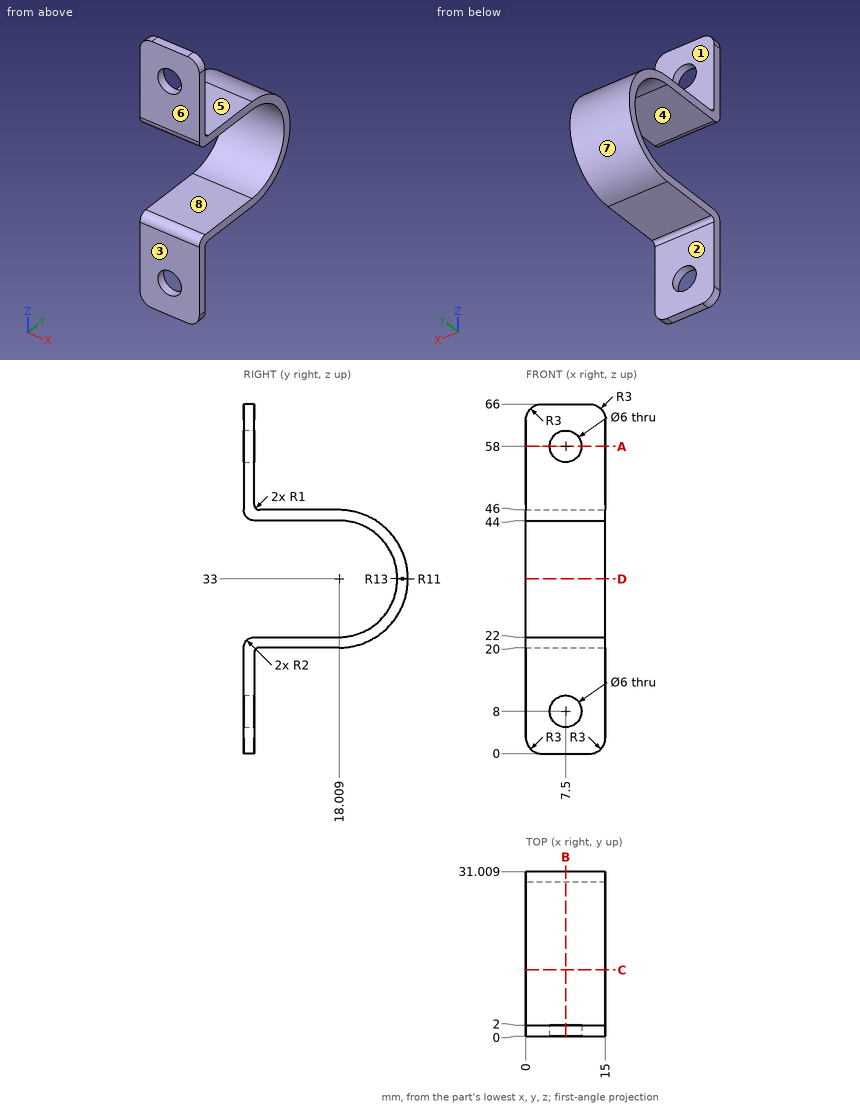
Study the drawing (mm; zero at the part's minimum x, y, z) and answer. A direction names the side the tool comes from. Round coordinates to 2 decimals unless told otherwise and drop trailing zeros. Order: outer loops, then holes, each group sorted by start corner. A loop starts at its lowest first (then second) coordinate and runs counter-clockwise, first axis right, second up. Notation, with made-up numbers: M 41.5,39 L 98.5,39 A30 ccw 98.5,61 Z; hole C -38.75,-40 d8. An arc over 180 degrees is marked long. One line per item, written item: value.
Q1. Flat-ended cylindrical pins translate along their axes: pin 1 (3 mm diameter, centred on x = 1.5, z = 57.5, fed in from +Y); pin 2 (1.5 mm diameter, centred on x = 4, y = 22.5, fed in from -Z); pin 3 (5 mm diameter, centred on x = 10, y = 17.5, fed in from -Z). Find the tip coordinate at first contact, or state that the pin passes through.
Derived:
pin 1: y = 2
pin 2: z = 20.55
pin 3: z = 20
Q2. For the marked faces 1, 2, 3 and 4, determine the directions among +Z, -Z, +X, -X, +Y, -Y from which every point of the face is accessible in a straight line to the end or side of a thin tool.
Derived:
face 1: +Z, +X, -X, +Y
face 2: -Z, +X, -X, +Y
face 3: +Z, -Z, +X, -X, -Y
face 4: +X, -X, -Y
Q3. Find section B-B on x = 7.5. Write down the section's boundary in (y, z), then the cut area to 3 significant figures.
Derived:
outline: M 0,0 L 2,0 L 2,5 L 0,5 Z; M 0,11 L 2,11 L 2,19 A1 cw 3,20 L 18.01,20 A13 ccw 18.01,46 L 3,46 A1 cw 2,47 L 2,55 L 0,55 L 0,46 A2 ccw 2,44 L 18.01,44 A11 cw 18.01,22 L 2,22 A2 ccw 0,20 Z; M 0,61 L 2,61 L 2,66 L 0,66 Z
area: 202 mm²
Q4. Determine the mould class of the marked faces 5, 6, 7 and 8 for opening direction Z: released by +Z, released by -Z, zero draft, split by the parting line, or undercut.
Derived:
face 5: released by +Z
face 6: zero draft
face 7: split by the parting line
face 8: undercut
Q5. Find section C-C on y = 12.5. Write down the section's boundary in (x, z).
Derived:
outline: M 0,20 L 15,20 L 15,22 L 0,22 Z; M 0,44 L 15,44 L 15,46 L 0,46 Z
Q6. Find section A-A on z = 58. Write down the section's boundary in (x, y).
Derived:
outline: M 0,0 L 4.5,0 L 4.5,2 L 0,2 Z; M 10.5,0 L 15,0 L 15,2 L 10.5,2 Z
Q7. Find section D-D on z = 33. Write down the section's boundary in (x, y), then the cut area to 3 significant figures.
Derived:
outline: M 0,29.01 L 15,29.01 L 15,31.01 L 0,31.01 Z
area: 30.0 mm²
Q8. Straight lines are drawn through the part: line 1 (Z direction, x = 5.25, y = 6); line 2 (Z direction, x = 7.5, y = 0.5) (1 decimal); line 3 (X direction, y = 1.6, z = 58). For each, find the intervals that lie inside material, in ascending order.
Derived:
line 1: 20 to 22, 44 to 46
line 2: 0 to 5, 11 to 21.3, 44.7 to 55, 61 to 66
line 3: 0 to 4.5, 10.5 to 15
